Read the model definition and answer for the solid it produces. Units are mm, in the model's axes. A direction names the side the tool comes from. Give positions to 0.01 mm unless a question says otherwise; leave off trailing zeros. Write each loop counter-clockwise with the first axis right and the second up, starting at its lowest first coordinate (ties: lowest second). Pieces come first, ordered by that corner, then holes. Notation, with made-up numbers: M 78,8 L 126,8 A28 cw 126,45 Z; hole C 54.25,89.5 d3. An arc over 180 degrees is marked long. Write each question's results on one line, items separated by ' | '. Start each with the question number.
```python
from build123d import *

# Parameters (mm, degrees)
SKETCH3_W = 0.254
SKETCH3_H = 0.508


with BuildPart() as part:
    # Sketch1 → Revolve1 (revolve)
    with BuildSketch(Plane.XY):
        Polygon((0, 0), (0, 3.175), (76.9874, 3.175), (76.9874, 11.19505), (98.3488, 11.19505), (98.3488, 0), align=None)
    revolve(axis=Axis((98.3488, 0, 0), (-1, 0, 0)))

    # Sketch2 → Revolve2 (revolve)
    with BuildSketch(Plane.XY):
        Polygon((-12.7, 0), (-12.7, 2.63398), (-12.15898, 3.175), (0, 3.175), (0, 0), align=None)
    revolve(axis=Axis((0, 0, 0), (-1, 0, 0)))

    # Sketch3 → Cut-Revolve1 (revolve, cut)
    with BuildSketch(Plane.XY):
        with Locations((-0.127, 3.175)):
            Rectangle(SKETCH3_W, SKETCH3_H)
    revolve(axis=Axis((0, 0, 0), (-1, 0, 0)), mode=Mode.SUBTRACT)


solid = part.part
```
Item 1: Straight lines are drawn through the part: line 1 (X direction, y = -9.5, z = 0); line 2 (Z direction, x = 89, y = -7); line 3 (Z direction, x = 81, y = -6). For each, find the intervals that lie inside material, in ascending order.
Item 2: Section A-A, the plane z = 0 is taken. Determine the outline of the cut face in (x, y) (3 decimals).
Item 3: Given P1, Ø4, axis at x = 47.5, y = -1, coming from the +Z side (3 decimals); P2, Ø1, axis at x = 45.5, z = 1, coming from the -Y side; P3, Ø1, axis at x = 54.5, y = -1.5, coming from the -Z side, each flat-ended and moving along its own axis, determine where each tip first touches the part or whether it passes through.
Item 4: For faces 1 (the flat face through (76.987, 3, 2)), 2 (the flat face through (-12.7, 0, 0)), determine the directions among +Z, -Z, +X, -X, +Y, -Y from which every point of the face is accessible in a straight line to the end or side of a thin tool.
Item 5: Section C-C, the plane x = 79.5 is taken. Determine the outline of the cut face in (y, z).
Item 6: Section D-D, the plane y = -7.5 is taken. Determine the outline of the cut face in (x, z).
Worked out:
1) line 1: x = 76.99 to 98.35 | line 2: z = -8.74 to 8.74 | line 3: z = -9.45 to 9.45
2) outline: M -12.7,-2.634 L -12.159,-3.175 L -0.254,-3.175 L -0.254,-2.921 L 0,-2.921 L 0,-3.175 L 76.987,-3.175 L 76.987,-11.195 L 98.349,-11.195 L 98.349,11.195 L 76.987,11.195 L 76.987,3.175 L 0,3.175 L 0,2.921 L -0.254,2.921 L -0.254,3.175 L -12.159,3.175 L -12.7,2.634 Z
3) P1: stops at z = 3.175 | P2: stops at y = -3.14 | P3: stops at z = -3.01
4) face 1: -X | face 2: +Z, -Z, -X, +Y, -Y
5) outline: C 0,0 d22.39
6) outline: M 76.99,-8.31 L 98.35,-8.31 L 98.35,8.31 L 76.99,8.31 Z
